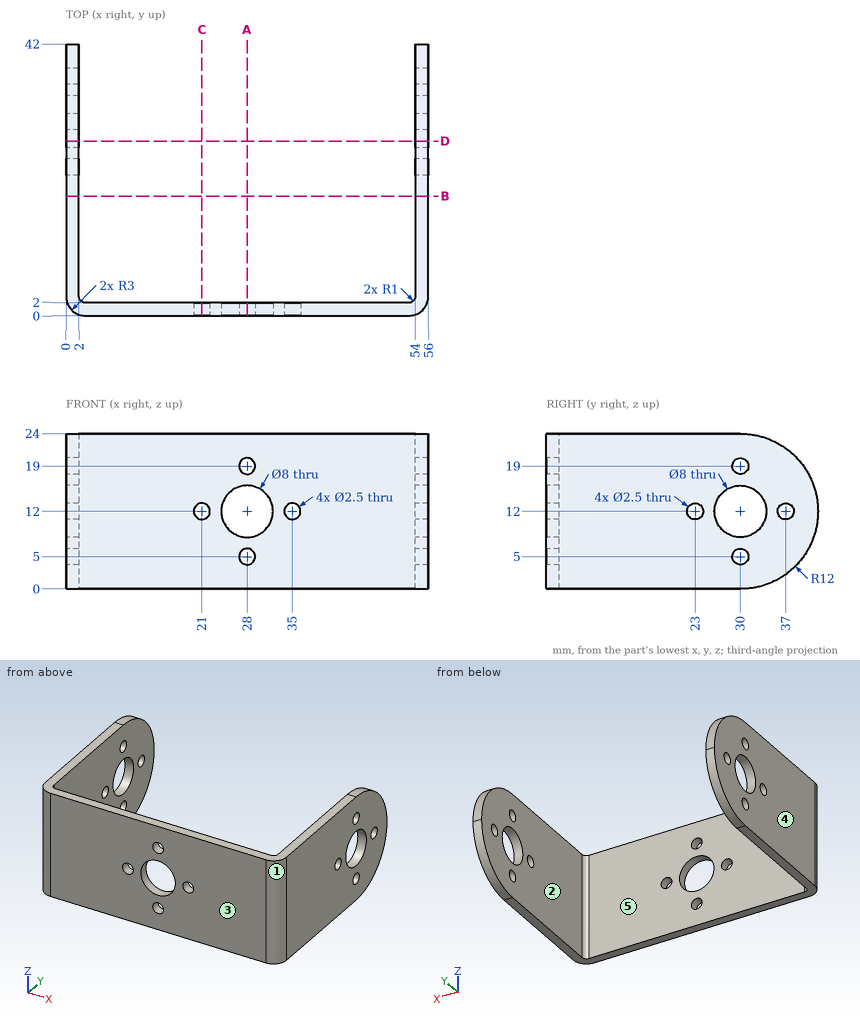
Drawing for the job (mm, zero at the part's lowest x, y, z). A direction names the side the tool comes from. Round coordinates to 2 decimals unless told otherwise and drop trailing zeros. Write each loop counter-clockwise with the first axis right and the second up, starting at its lowest first coordinate (ties: lowest second). Pieces come first, ordered by that corner, then holes. Notation, with made-up numbers: (-31.75, 61.25) - (4.25, 61.25) arc R28 cw to (4.25, 94.25) - close; hole circle Ø4 at (51, 86.25). An arc over 180 degrees is marked (long way). Write item = value, one per line. Start each with the question number.
Q1. Which spindle directions (+Z, -Z, +X, -X, +Y, -Y) get a long thin tool onto all of the face, cutting with end or side? Do the marked faces 1 and 2. Say none if no direction does.
Q2. Probe L1, parallel to X at y = 35, z = 7; L2, parallel to Z at x = 28, y = 1.6; L3, parallel to Y at x = 6.5, z = 12.5. List the from-to ranges inside material, lowest first. Write a range as from..to.
Q3. Band-saw the part on C-C (x = 21). Give the cut face in (y, z), then the cut area to 3 significant figures.
Q4. Band-saw the part on D-D (y = 27). Give the cut face in (x, z).
Q5. Band-saw the part on A-A (x = 28). Give the cut face in (y, z), then the cut area to 3 significant figures.
Q6. Mould opens along X. For the marked faces 3, 4 and 5 say: pulls with the +X half, pulls with the -X half, needs draft (parallel to the pull), parting line crosses it, or undercut.
Q7. Drop a flat-ended pin along its axis: pin 1 (4 mm diameter, centred on x = 11.5, z = 9.5, fed in from +Y). Give the stop position or say it passes through.
Q8. Band-saw the part on B-B (y = 18.5). Give the cut face in (x, z).
Answers below:
q1.face_1 = +Z, -Z, +X, -Y
q1.face_2 = +Z, -Z, +Y
q2.L1 = 0..2, 54..56
q2.L2 = 0..3.75, 6.25..8, 16..17.75, 20.25..24
q2.L3 = 0..2
q3.outline = (0, 0) - (2, 0) - (2, 10.75) - (0, 10.75) - close; (0, 13.25) - (2, 13.25) - (2, 24) - (0, 24) - close
q3.area = 43.0 mm2
q4.outline = (0, 0) - (2, 0) - (2, 9.35) - (0, 9.35) - close; (0, 14.65) - (2, 14.65) - (2, 24) - (0, 24) - close; (54, 0) - (56, 0) - (56, 9.35) - (54, 9.35) - close; (54, 14.65) - (56, 14.65) - (56, 24) - (54, 24) - close
q5.outline = (0, 0) - (2, 0) - (2, 3.75) - (0, 3.75) - close; (0, 6.25) - (2, 6.25) - (2, 8) - (0, 8) - close; (0, 16) - (2, 16) - (2, 17.75) - (0, 17.75) - close; (0, 20.25) - (2, 20.25) - (2, 24) - (0, 24) - close
q5.area = 22.0 mm2
q6.face_3 = needs draft
q6.face_4 = pulls with the -X half
q6.face_5 = undercut
q7.pin_1 = 2
q8.outline = (0, 0) - (2, 0) - (2, 24) - (0, 24) - close; (54, 0) - (56, 0) - (56, 24) - (54, 24) - close
